Verification items for this drawing (mm, ordinates from the low corner). Round coordinates to 2 decimals unless told otherwise and drop trailing zeros. Write each loop counter-clockwise with the first axis right and the second up, starting at its lowest first coordinate (ties: lowest second). Pieces come first, ordered by that corner, then holes. Notation, with made-up numbers: (31.5, 57.5) -> (90.5, 57.5) arc R23 cw to (90.5, 68.5) -> close; hole circle Ø1 at (72, 38). An arc over 180 degrees is marked (long way). One line per item, written item: value.
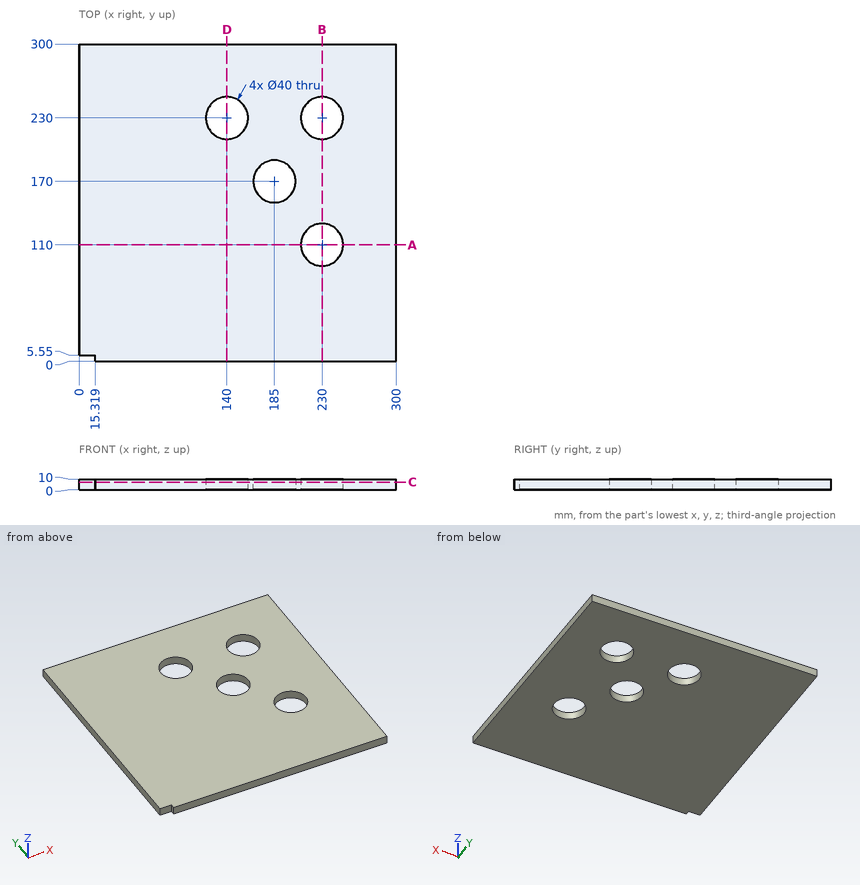
Item 1: Sectioned sample at A-A (y = 110). Enter the section's corners in (x, z).
Result set:
outline: (0, 0) -> (210, 0) -> (210, 10) -> (0, 10) -> close; (250, 0) -> (300, 0) -> (300, 10) -> (250, 10) -> close
Item 2: Material ranges on line 1 along Y through (x, z) = (230, 4.75); line 2 along X through (y, z) = (186, 4); line 3 along X through (y, z) = (173, 3), recorded low to high.
Result set:
line 1: 0 to 90, 130 to 210, 250 to 300
line 2: 0 to 173, 197 to 300
line 3: 0 to 165.23, 204.77 to 300
Item 3: Sectioned sample at C-C (z = 7). Enter the section's corners in (x, y), then the cut area to 3 significant figures.
Result set:
outline: (0, 5.55) -> (15.32, 5.55) -> (15.32, 0) -> (300, 0) -> (300, 300) -> (0, 300) -> close; hole circle Ø40 at (140, 230); hole circle Ø40 at (185, 170); hole circle Ø40 at (230, 110); hole circle Ø40 at (230, 230)
area: 84,900 mm^2
Item 4: Depth check by flat-ended pin: pin 1 (5 mm diameter, centred on x = 6, z = 4.5, fed in from -Y); pin 2 (6 mm diameter, centred on y = 1.5, z = 7, fed in from -X). Enter the tip coordinate at first touch or a pass-through.
Result set:
pin 1: y = 5.55
pin 2: x = 15.32
Item 5: Sectioned sample at B-B (x = 230). Enter the section's corners in (y, z).
Result set:
outline: (0, 0) -> (90, 0) -> (90, 10) -> (0, 10) -> close; (130, 0) -> (210, 0) -> (210, 10) -> (130, 10) -> close; (250, 0) -> (300, 0) -> (300, 10) -> (250, 10) -> close
